```python
from build123d import *

# Parameters (mm, degrees)
SKETCH1_W            = 25
SKETCH1_H            = 8
BOSS_EXTRUDE1_DEPTH  = 15
SKETCH3_W            = 6.25
SKETCH3_H            = 4
CUT_EXTRUDE1_DEPTH   = 12
M4_CLEARANCE_HOLE1_D = 4.5


with BuildPart() as part:
    # Sketch1 → Boss-Extrude1 (new, symmetric)
    with BuildSketch(Plane.XY):
        Rectangle(SKETCH1_W, SKETCH1_H)
    extrude(amount=BOSS_EXTRUDE1_DEPTH, both=True)

    # Sketch3 → Cut-Extrude1 (cut)
    with BuildSketch(Plane(origin=(0, 0, -12), x_dir=(-1, 0, 0), z_dir=(0, 0, -1))):
        with Locations((0, 2)):
            Rectangle(SKETCH3_W, SKETCH3_H)
    extrude(amount=-CUT_EXTRUDE1_DEPTH, mode=Mode.SUBTRACT)

    # M4 Clearance Hole1 (through all)
    with Locations(Plane(origin=(0, -4, 0), x_dir=(-1, 0, 0), z_dir=(0, -1, 0))):
        with Locations((0, -7.5)):
            Hole(M4_CLEARANCE_HOLE1_D / 2)


solid = part.part
```
CAD build for the part. Positions are in the model's coordinates, mm. A direction names the side the tool comes from. Round coordinates to 2 decimals unless told otherwise and drop trailing zeros. Order: outer loops, then holes, each group sorted by start corner. A loop starts at its lowest first (then second) coordinate and runs counter-clockwise, first axis right, second up. Notation, with made-up numbers: (-39.5, 34) -> (15.5, 34) arc R33 ccw to (15.5, 68) -> close; hole circle Ø1 at (-28, -37.5). An arc over 180 degrees is marked (long way). One line per question, with ' | ' between items.
Q1. Drop a flat-ended pin along its axis: pin 1 (7 mm diameter, centred on x = 0, z = -4.5, fed in from +Y). Give the stop position or say it passes through.
Completed:
pin 1: stops at y = 4
Q2. Two-plate mould, pull along X, no slides. Class faces 3 (the flat face through (12.5, 0, 0)), 4 (the flat face through (0, -4, 0)), 5 (the cylindrical face through (-0.29, 0.06, 5.27)): released by +X, released by -X, zero draft, split by the parting line, or undercut.
Completed:
face 3: released by +X | face 4: zero draft | face 5: undercut
Q3. Slice it at D-D (y = -2.25). Write the cut outline in (x, z), then the cut area to 3 significant figures.
Completed:
outline: (-12.5, -15) -> (12.5, -15) -> (12.5, 15) -> (-12.5, 15) -> close; hole circle Ø4.5 at (0, 7.5) | area: 734 mm^2
Q4. Probe probe 1 along Z at (x, y) = (0, 0.5); probe 2 along Z at (x, y) = (0, -1); probe 3 along Z at (x, y) = (1.25, 2). List the from-to ranges inside material, lowest first.
Completed:
probe 1: z = -15 to -12, 0 to 5.25, 9.75 to 15 | probe 2: z = -15 to 5.25, 9.75 to 15 | probe 3: z = -15 to -12, 0 to 5.63, 9.37 to 15
Q5. Slice it at B-B (z = 7.5). Write the cut outline in (x, y).
Completed:
outline: (-12.5, -4) -> (-2.25, -4) -> (-2.25, 4) -> (-12.5, 4) -> close; (2.25, -4) -> (12.5, -4) -> (12.5, 4) -> (2.25, 4) -> close
Q6. Slice it at C-C (y = 1). Write the cut outline in (x, z) (3 decimals).
Completed:
outline: (-12.5, -15) -> (12.5, -15) -> (12.5, 15) -> (-12.5, 15) -> close; hole (-3.125, -12) -> (3.125, -12) -> (3.125, 0) -> (-3.125, 0) -> close; hole circle Ø4.5 at (0, 7.5)
Q7. Slice it at A-A (x = 0). Write the cut outline in (y, z).
Completed:
outline: (-4, -15) -> (4, -15) -> (4, -12) -> (0, -12) -> (0, 0) -> (4, 0) -> (4, 5.25) -> (-4, 5.25) -> close; (-4, 9.75) -> (4, 9.75) -> (4, 15) -> (-4, 15) -> close
Q8. Which spindle directions (+Z, -Z, +X, -X, +Y, -Y) get a long thin tool onto all of the face, cutting with end or side? Do faces 1 (the flat face through (-3.125, 2, -6)), 2 (the flat face through (0, 0, 15)). Say none if no direction does.
Completed:
face 1: +Y | face 2: +Z, +X, -X, +Y, -Y
